Geometry: final body of the model. Coordinates: model frame, mm. A direction names the side the tool comes from. Coordinates: 2 decimals unless noted, no trailing zeros. Write each loop counter-clockwise with the first axis right and the second up, starting at its lowest first coordinate (ties: lowest second). Pieces come first, ordered by that corner, then holes. Notation, with made-up numbers: (80.25, 89) - (132.25, 89) arc R25 cw to (132.25, 118) - close; hole circle Ø10 at (-40, -26.5). An arc over 180 degrees is marked (long way). Answer as a JSON object with one key per item and string values. Group by question number.
Item 1: Line query: line 1 along Z through (x, y) = (5, 15); line 2 along Z through (x, y) = (-5, 1.75); line 3 along Y through (x, z) = (-12, 11.6). Output: solid intervals per line, ascending. Write a range as from..to.
Item 2: Set-up query: faces 1 (the flat face through (12, 3, 10)), 2 (the cylindrical face through (-11, 2.5, -12.5)), 3 (the flat face through (11.4, 5, 0)), 4 (the cylindrical face through (-5.026, 7.535, 0.079)), 5 (the cylindrical face through (16.085, 13.549, 4.596)). Return all of +Z, -Z, +X, -X, +Y, -Y with unobstructed straight access to the full face (end or side cutting, diameter ignored); none if empty.
Item 3: Section B-B on x = -9. Return loops of the section in (y, z).
Item 4: Section A-A on y = 2.5. Return loops of the section in (x, z).
Item 5: Section C-C on z = 3. Return loops of the section in (x, y).
Item 6: First-contact query: pin 1 Ø1.5 at (x, y) = (-5.5, 6) entering from +Z; pin 2 Ø4 at (x, y) = (-9.5, 13.5) entering from -Z; pin 3 Ø0.8 at (x, y) = (-1, 6.5) entering from -Z (3 decimals); pin 4 Ø1.6 at (x, y) = (-12, 3) entering from +Z. Flat tips, straight axial feed; report the tip coordinate or a pass-through.
Item 7: Mould query, pull axis Y, two halves, no side actions, for faces 6 (the flat face through (7, 17, 12)), 7 (the flat face through (-12, 3, -10)), 8 (the flat face through (-1, 8, -3.571)). Classes: pulls with the +Y half, pulls with the -Y half, needs draft (parallel to the pull), parting line crosses it, or undercut.
Item 8: Section D-D on y = 11.75. Return loops of the section in (x, z), and give its area (3 significant figures).
```python
from build123d import *

# Parameters (mm, degrees)
SKETCH_1_W               = 36
SKETCH_1_H               = 30
EXTRUDE_1_DEPTH          = 5
SKETCH_2_R               = 14.5
EXTRUDE_2_DEPTH          = 17
SKETCH_4_W               = 33
SKETCH_4_H               = 12
CUT_EXTRUDE_2_DEPTH      = 2
SKETCH_8_R               = 1
CUT_EXTRUDE_6_DEPTH      = 3
SKETCH_5_W               = 23.5
SKETCH_5_H               = 12
CUT_EXTRUDE_3_DEPTH      = 3
CUT_EXTRUDE_3_DEPTH_BACK = 3
SKETCH_3_R               = 12
CUT_EXTRUDE_1_DEPTH      = 7
SKETCH_6_R               = 6
CUT_EXTRUDE_4_DEPTH      = 5
CUT_EXTRUDE_5_DEPTH      = 5
SKETCH_9_R               = 1
CUT_EXTRUDE_7_DEPTH      = 5


with BuildPart() as part:
    # 草图1 → 凸台-拉伸1 (new body)
    with BuildSketch(Plane(origin=(0, 0, 0), x_dir=(1, 0, 0), z_dir=(0, 1, 0))):
        Rectangle(SKETCH_1_W, SKETCH_1_H)
    extrude(amount=EXTRUDE_1_DEPTH)

    # 草图2 → 凸台-拉伸2 (add)
    with BuildSketch(Plane.XZ):
        with Locations((5, 0)):
            Circle(SKETCH_2_R)
    extrude(amount=-EXTRUDE_2_DEPTH)

    # 草图4 → 切除-拉伸2 (cut)
    with BuildSketch(Plane.XZ):
        Rectangle(SKETCH_4_W, SKETCH_4_H)
    extrude(amount=-CUT_EXTRUDE_2_DEPTH, mode=Mode.SUBTRACT)

    # 草图8 → 切除-拉伸6 (cut)
    with BuildSketch(Plane.XZ.offset(-2)):
        with Locations((14, 0)):
            Circle(SKETCH_8_R)
        with Locations((-14, 0)):
            Circle(SKETCH_8_R)
    extrude(amount=-CUT_EXTRUDE_6_DEPTH, mode=Mode.SUBTRACT)

    # 草图5 → 切除-拉伸3 (cut, two sides)
    with BuildSketch(Plane.XZ.offset(-2)) as cut_extrude_3_sk:
        Rectangle(SKETCH_5_W, SKETCH_5_H)
    extrude(amount=CUT_EXTRUDE_3_DEPTH, mode=Mode.SUBTRACT)
    extrude(cut_extrude_3_sk.sketch, amount=-CUT_EXTRUDE_3_DEPTH_BACK, mode=Mode.SUBTRACT)

    # 草图3 → 切除-拉伸1 (cut)
    with BuildSketch(Plane(origin=(0, 17, 0), x_dir=(1, 0, 0), z_dir=(0, 1, 0))):
        with Locations((5, 0)):
            Circle(SKETCH_3_R)
    extrude(amount=-CUT_EXTRUDE_1_DEPTH, mode=Mode.SUBTRACT)

    # 草图6 → 切除-拉伸4 (cut)
    with BuildSketch(Plane(origin=(0, 10, 0), x_dir=(1, 0, 0), z_dir=(0, 1, 0))):
        with Locations((5, 0)):
            Circle(SKETCH_6_R)
    extrude(amount=-CUT_EXTRUDE_4_DEPTH, mode=Mode.SUBTRACT)

    # 草图7 → 切除-拉伸5 (cut)
    with BuildSketch(Plane(origin=(0, 10, 0), x_dir=(1, 0, 0), z_dir=(0, 1, 0))):
        with BuildLine():
            Line((-1.455492537, 3.570915288), (2.115422752, 3.570915288))
            Line((2.115422752, 3.570915288), (2.115422752, -3.570915288))
            Line((2.115422752, -3.570915288), (-1.455492537, -3.570915288))
            ThreePointArc((-1.455492537, -3.570915288), (-5.026407825, 0), (-1.455492537, 3.570915288))
        make_face()
    extrude(amount=-CUT_EXTRUDE_5_DEPTH, mode=Mode.SUBTRACT)

    # 草图9 → 切除-拉伸7 (cut)
    with BuildSketch(Plane(origin=(0, 0, -15), x_dir=(-1, 0, 0), z_dir=(0, 0, -1))):
        with Locations((12, 2.5)):
            Circle(SKETCH_9_R)
        with Locations((-12, 2.5)):
            Circle(SKETCH_9_R)
    cut_extrude_7 = extrude(amount=-CUT_EXTRUDE_7_DEPTH, mode=Mode.SUBTRACT)

    # 镜向1: 切除-拉伸7 across plane
    add(cut_extrude_7.mirror(Plane.XY), mode=Mode.SUBTRACT)


solid = part.part
```
Checks:
{
 "1": {"line 1": "-14.5..-12, 12..14.5", "line 2": "-15..-6, 6..15", "line 3": "0..1.5, 3.5..5"},
 "2": {"face 1": "+Z", "face 2": "-Z", "face 3": "-Y", "face 4": "+Y, -Y", "face 5": "+Y"},
 "3": {"outline": "(0, -15) - (5, -15) - (5, -6) - (0, -6) - close; (0, 6) - (5, 6) - (5, 15) - (0, 15) - close; (5, -3.77) - (17, -3.77) - (17, 3.77) - (5, 3.77) - close"},
 "4": {"outline": "(-18, -15) - (-13, -15) - (-13, -10) - (-11, -10) - (-11, -15) - (11, -15) - (11, -10) - (13, -10) - (13, -15) - (18, -15) - (18, -6.42) arc R14.5 ccw to (18, 6.42) - (18, 15) - (13, 15) - (13, 10) - (11, 10) - (11, 15) - (-11, 15) - (-11, 10) - (-13, 10) - (-13, 15) - (-18, 15) - close; hole circle Ø2 at (-14, 0); hole (-11.75, -6) - (11.75, -6) - (11.75, 6) - (-11.75, 6) - close; hole circle Ø2 at (14, 0)"},
 "5": {"outline": "(-18, 0) - (-16.5, 0) - (-16.5, 2) - (-11.75, 2) - (-11.75, 5) - (-18, 5) - close; (-9.19, 5) - (-3.39, 5) - (-3.39, 10) - (-6.62, 10) - (-6.62, 17) - (-9.19, 17) - close; (10.2, 5) - (11.75, 5) - (11.75, 2) - (16.5, 2) - (16.5, 0) - (19.19, 0) - (19.19, 17) - (16.62, 17) - (16.62, 10) - (10.2, 10) - close"},
 "6": {"pin 1": "z = 10.73", "pin 2": "z = -7.35", "pin 3": "z = -13.375", "pin 4": "z = 15"},
 "7": {"face 6": "pulls with the +Y half", "face 7": "undercut", "face 8": "needs draft"},
 "8": {"outline": "circle Ø29 at (5, 0); hole circle Ø24 at (5, 0)", "area": "208 mm^2"}
}
